Input: part model. Units: mm. Frame: model coordinates. Face numbers are marked on the shaded views. A direction names the side the tool comes from. Give positions to 0.01 mm unless a question says otherwise; leave off trailing zeros. Loops run counter-clockwise (first coordinate to the right, second up) from the corner with the lowest first, then second, coordinate; pieces in that order, holes last.
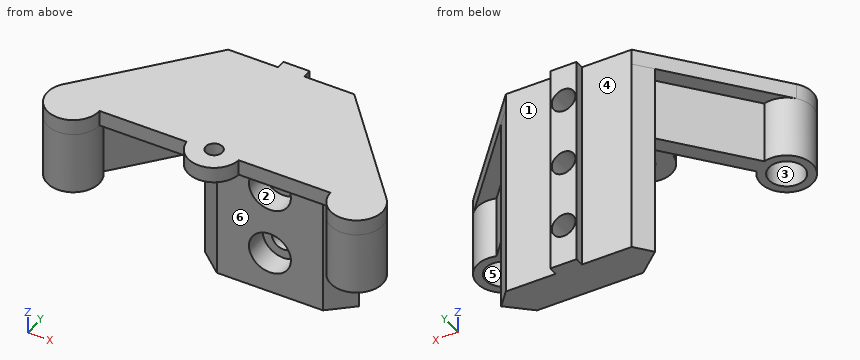
from build123d import *

# Parameters (mm, degrees)
BOSS_EXTRUDE1_DEPTH = 3
SKETCH2_R           = 3.39
BOSS_EXTRUDE2_DEPTH = 12
BOSS_EXTRUDE3_DEPTH = 26
SKETCH7_W           = 5
SKETCH7_H           = 1.7
BOSS_EXTRUDE5_DEPTH = 41
SKETCH4_R           = 2.25
CUT_EXTRUDE1_DEPTH  = 13
SKETCH8_R           = 4
CUT_EXTRUDE3_DEPTH  = 4.5
LPATTERN1_COUNT     = 3
LPATTERN1_PITCH     = 13
SKETCH5_R           = 5
BOSS_EXTRUDE4_DEPTH = 3
SKETCH6_R           = 1.6
CUT_EXTRUDE2_DEPTH  = 3


with BuildPart() as part:
    # Sketch1 → Boss-Extrude1 (new body)
    with BuildSketch(Plane.XY):
        with BuildLine():
            Line((-22, 0), (22, 0))
            ThreePointArc((22, 0), (28.74444357, -4.685820806), (30.782766652, 3.269659991))
            Line((30.782766652, 3.269659991), (12, 25))
            Line((12, 25), (-12, 25))
            Line((-12, 25), (-30.782766652, 3.269659991))
            ThreePointArc((-30.782766652, 3.269659991), (-28.74444357, -4.685820806), (-22, 0))
        make_face()
    extrude(amount=-BOSS_EXTRUDE1_DEPTH)

    # Sketch2 → Boss-Extrude2 (add)
    with BuildSketch(Plane(origin=(0, 0, -3), x_dir=(-1, 0, 0), z_dir=(0, 0, -1))):
        with BuildLine():
            Line((10.11979413, 18), (-10.11979413, 18))
            Line((-10.11979413, 18), (-23.039847225, 3.052407247))
            ThreePointArc((-23.039847225, 3.052407247), (-29.854865308, -4.104843977), (-25.51641378, 4.7748269))
            Line((-25.51641378, 4.7748269), (-12.389454122, 19.961795995))
            Line((-12.389454122, 19.961795995), (-14.659114113, 21.923591989))
            Line((-14.659114113, 21.923591989), (-12, 25))
            Line((-12, 25), (12, 25))
            Line((12, 25), (14.659114113, 21.923591989))
            Line((14.659114113, 21.923591989), (12.389454122, 19.961795995))
            Line((12.389454122, 19.961795995), (25.51641378, 4.7748269))
            ThreePointArc((25.51641378, 4.7748269), (29.854865308, -4.104843977), (23.039847225, 3.052407247))
            Line((23.039847225, 3.052407247), (10.11979413, 18))
        make_face()
        with Locations((27, 0)):
            Circle(SKETCH2_R, mode=Mode.SUBTRACT)
        with Locations((-27, 0)):
            Circle(SKETCH2_R, mode=Mode.SUBTRACT)
    extrude(amount=BOSS_EXTRUDE2_DEPTH)

    # Sketch3 → Boss-Extrude3 (add)
    with BuildSketch(Plane(origin=(0, 0, -15), x_dir=(-1, 0, 0), z_dir=(0, 0, -1))):
        Polygon((14.659114113, 21.923591989), (10.11979413, 18), (-10.11979413, 18), (-14.659114113, 21.923591989), (-12, 25), (12, 25), align=None)
    extrude(amount=BOSS_EXTRUDE3_DEPTH)

    # Sketch7 → Boss-Extrude5 (add)
    with BuildSketch(Plane(origin=(0, 0, -41), x_dir=(-1, 0, 0), z_dir=(0, 0, -1))):
        with Locations((0, 25.85)):
            Rectangle(SKETCH7_W, SKETCH7_H)
    extrude(amount=-BOSS_EXTRUDE5_DEPTH)

    # Sketch4 → Cut-Extrude1 (cut, symmetric)
    with BuildSketch(Plane(origin=(0, 25, 0), x_dir=(-1, 0, 0), z_dir=(0, 1, 0))):
        with Locations((0, -33)):
            Circle(SKETCH4_R)
        with Locations((0, -20)):
            Circle(SKETCH4_R)
        with Locations((0, -7)):
            Circle(SKETCH4_R)
    extrude(amount=CUT_EXTRUDE1_DEPTH, both=True, mode=Mode.SUBTRACT)

    # Sketch8 → Cut-Extrude3 (cut)
    with BuildSketch(Plane(origin=(0, 18, 0), x_dir=(-1, 0, 0), z_dir=(0, -1, 0))):
        with Locations((0, 33)):
            Circle(SKETCH8_R)
    cut_extrude3 = extrude(amount=-CUT_EXTRUDE3_DEPTH, mode=Mode.SUBTRACT)

    # LPattern1: Cut-Extrude3 ×3
    with Locations(*[(0, 0, i * LPATTERN1_PITCH) for i in range(1, LPATTERN1_COUNT)]):
        add(cut_extrude3, mode=Mode.SUBTRACT)

    # Sketch5 → Boss-Extrude4 (add)
    with BuildSketch(Plane.XY):
        with Locations((-0.455639948, 0.495332174)):
            Circle(SKETCH5_R)
    extrude(amount=-BOSS_EXTRUDE4_DEPTH)

    # Sketch6 → Cut-Extrude2 (cut)
    with BuildSketch(Plane.XY):
        with Locations((-0.455639948, 0.495332174)):
            Circle(SKETCH6_R)
    extrude(amount=-CUT_EXTRUDE2_DEPTH, mode=Mode.SUBTRACT)


solid = part.part
(1) Cut plane D-D (y = 7). Return the cut outline in (x, z), and give its area (3 significant figures).
Values follow:
outline: (-27.56, -3) - (-23.59, -3) - (-23.59, -15) - (-19.63, -15) - (-19.63, -3) - (19.63, -3) - (19.63, -15) - (23.59, -15) - (23.59, -3) - (27.56, -3) - (27.56, 0) - (-27.56, 0) - close
area: 261 mm2
(2) Cut plane C-C (x = 27). Return the cut outline in (y, z).
Values follow:
outline: (-5, -15) - (-3.39, -15) - (-3.39, -3) - (3.39, -3) - (3.39, -15) - (5, -15) - (5, -3) - (7.65, -3) - (7.65, 0) - (-5, 0) - close
(3) Cut plane A-A (z = -7). Return the cut outline in (x, y).
Values follow:
outline: (-25.52, 4.77) arc R5 ccw (long way) to (-23.04, 3.05) - (-10.12, 18) - (-4, 18) - (-4, 22.5) - (-2.25, 22.5) - (-2.25, 26.7) - (-2.5, 26.7) - (-2.5, 25) - (-12, 25) - (-14.66, 21.92) - (-12.39, 19.96) - close; (2.25, 22.5) - (4, 22.5) - (4, 18) - (10.12, 18) - (23.04, 3.05) arc R5 ccw (long way) to (25.52, 4.77) - (12.39, 19.96) - (14.66, 21.92) - (12, 25) - (2.5, 25) - (2.5, 26.7) - (2.25, 26.7) - close; hole circle Ø6.78 at (-27, 0); hole circle Ø6.78 at (27, 0)
(4) Pin query (flat end, axial travel): pin 1 Ø2 at (x, y) = (15.5, 3.5) entering from -Z; pin 2 Ø5 at (x, z) = (-11.5, -24) entering from -Y; pin 3 Ø6.5 at (x, z) = (0, -20) entering from +Y; pin 4 Ø13 at (x, z) = (0, -7) entering from -Y. Return the tip coordinate at first contact, or that it passes through.
Values follow:
pin 1: stops at z = -3
pin 2: stops at y = 18
pin 3: stops at y = 26.7
pin 4: stops at y = -4.5
(5) Cut plane B-B (z = -33). Return the cut outline in (x, y).
Values follow:
outline: (-14.66, 21.92) - (-10.12, 18) - (-4, 18) - (-4, 22.5) - (-2.25, 22.5) - (-2.25, 26.7) - (-2.5, 26.7) - (-2.5, 25) - (-12, 25) - close; (2.25, 22.5) - (4, 22.5) - (4, 18) - (10.12, 18) - (14.66, 21.92) - (12, 25) - (2.5, 25) - (2.5, 26.7) - (2.25, 26.7) - close
(6) Mould query, pull axis X, two halves, no side actions, for the marked faces 4, 5 and 6. Classes: +X half, -X half, draft (parallel to the pull), parting line (faces both ways), or undercut.
Values follow:
face 4: draft
face 5: undercut
face 6: undercut
(7) Reachability of the marked faces 1, 2 and 3 from +Z, -Z, +X, -X, +Y, -Y: full face, straight path, thin tool, end or side. Return the list, or none.
Values follow:
face 1: +Z, -Z, +X, +Y
face 2: -Y
face 3: -Z
(8) Ray query, probe 1 along Z at (x, y) = (0, 21.2); probe 2 along Z at (x, y) = (0, 23); probe 3 along X at (y, z) = (25.25, -20). Return the intervals inside material, ascending.
Values follow:
probe 1: z = -41 to -37, -29 to -24, -16 to -11, -3 to 0
probe 2: z = -41 to -35.25, -30.75 to -22.25, -17.75 to -9.25, -4.75 to 0
probe 3: x = -2.5 to -2.25, 2.25 to 2.5
